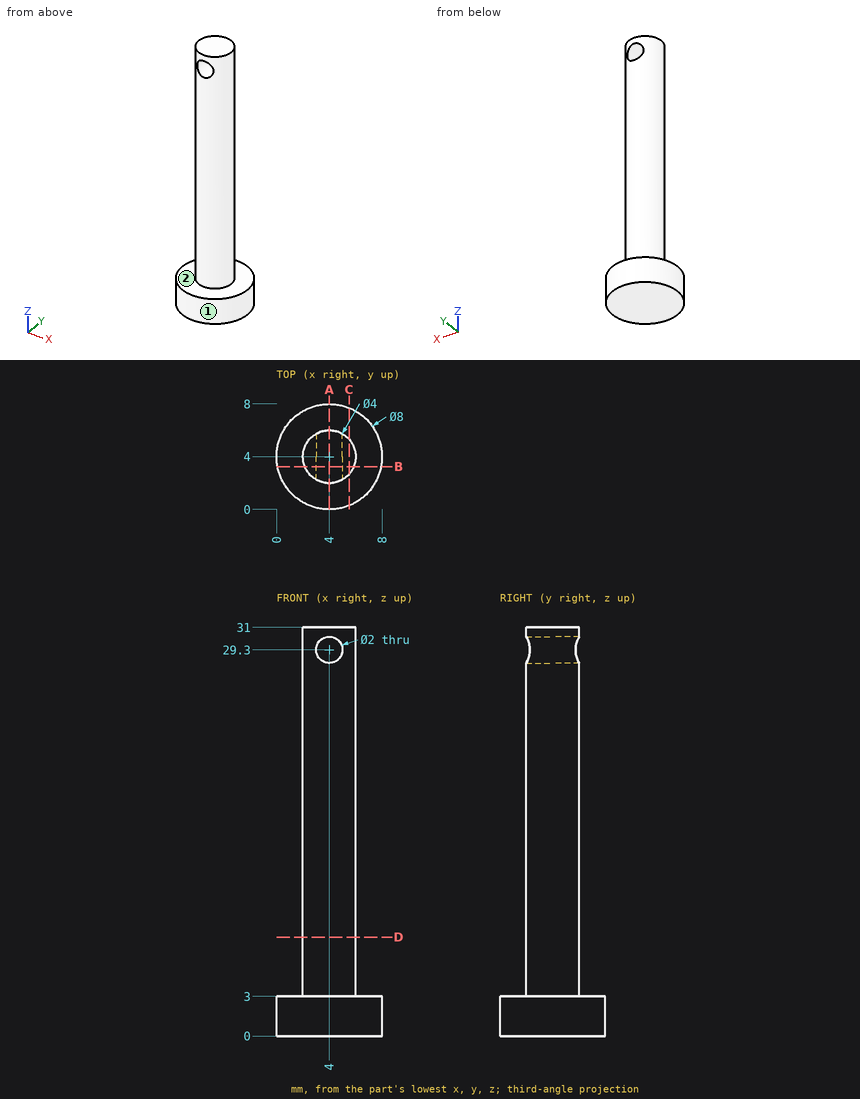
Check sheet for the drawn part. Datum: minimum x, y, z corner. Units: mm. A direction names the side the tool comes from. Round coordinates to 2 decimals unless told otherwise and drop trailing zeros. Write each loop counter-clockwise with the first axis right and the second up, starting at its lowest first coordinate (ties: lowest second). Pieces come first, ordered by that corner, then holes. Notation, with made-up numbers: (54.25, 67) - (80.25, 67) arc R9 ccw to (80.25, 73) - close; hole circle Ø6 at (49.5, -36.5). An arc over 180 degrees is marked (long way). Return JSON: item names as keys, results as strings.
Q1. Cross-section at B-B (y = 3.25). Record the boundary of the cut face in (x, z).
Returned:
{"outline": "(0.07, 0) - (7.93, 0) - (7.93, 3) - (5.85, 3) - (5.85, 31) - (2.15, 31) - (2.15, 3) - (0.07, 3) - close; hole circle Ø2 at (4, 29.3)"}
Q2. Cross-section at C-C (x = 5.5). Record the boundary of the cut face in (y, z).
Returned:
{"outline": "(0.29, 0) - (7.71, 0) - (7.71, 3) - (5.32, 3) - (5.32, 31) - (2.68, 31) - (2.68, 3) - (0.29, 3) - close"}
Q3. Scan lines: L1, parallel to Z at x = 4, y = 3.2; L2, parallel to Z at x = 1.75, y = 0.75; L3, parallel to X at y = 2.45, z = 29.3. Record each from-to range of solid material in increasing order. Write a range as from..to.
Returned:
{"L1": "z = 0..28.3, 30.3..31", "L2": "z = 0..3", "L3": "x = 2.74..3, 5..5.26"}
Q4. Access from +Z, -Z, +X, -X, +Y, -Y to the whole of each face (thin tool, end or side, straight path). Record for the marked faces 1 and 2.
Returned:
{"face 1": "+Z, -Z", "face 2": "+Z"}
Q5. Cross-section at A-A (x = 4). Record the boundary of the cut face in (y, z), then the cut area to 3 significant figures.
Returned:
{"outline": "(0, 0) - (8, 0) - (8, 3) - (6, 3) - (6, 28.3) - (2, 28.3) - (2, 3) - (0, 3) - close; (2, 30.3) - (6, 30.3) - (6, 31) - (2, 31) - close", "area": "128 mm²"}
Q6. Cross-section at D-D (z = 7.5). Record the boundary of the cut face in (x, y).
Returned:
{"outline": "circle Ø4 at (4, 4)"}
Q7. Depth check by flat-ended pin: P1, Ø2, axis at x = 4, z = 9, coming from the +Y side; P2, Ø3, axis at y = 3.5, z = 18, coming from the +X side; P3, Ø1.5, axis at x = 5.5, y = 7, coming from the +Z side. Enter the tip coordinate at first touch or a pass-through.
Returned:
{"P1": "stops at y = 6", "P2": "stops at x = 6", "P3": "stops at z = 3"}
